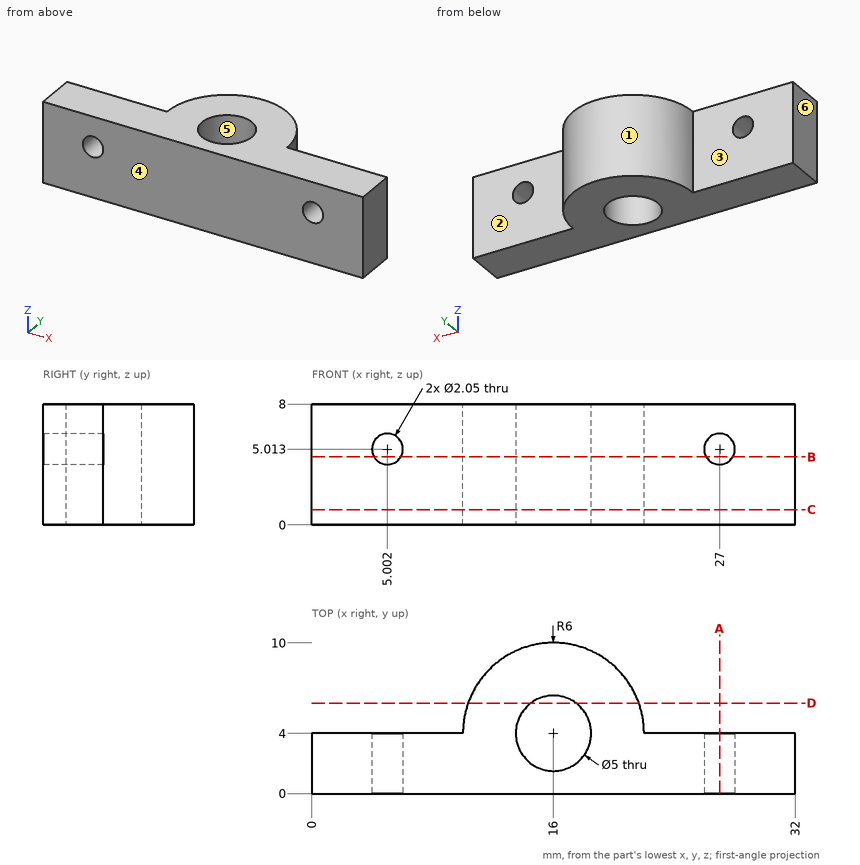
The figure shows three views and two pictorial views of one solid part (mm, origin at its lowest corner). Answer the questions. A direction names the side the tool comes from. Coordinates: 2 decimals unless noted, no trailing zeros. Loops run counter-clockwise (first coordinate to the right, second up) from the corner with the lowest first, then second, coordinate; pieces in that order, holes last. Notation, with made-up numbers: (-25.75, -12) - (4.25, -12) arc R21 cw to (4.25, 3) - close; hole circle Ø4 at (86, -25). An arc over 180 degrees is marked (long way). Write item = value, one per line.
1) Determine the mould class of the marked faces 4, 5 and 6 for opening direction X: pulls with the +X half, pulls with the -X half, needs draft (parallel to the pull), parting line crosses it, or undercut.
Responses:
face_4 = needs draft
face_5 = undercut
face_6 = pulls with the -X half
2) Section D-D (y = 6) is taken. Determine the outline of the cut face in (x, z).
Responses:
outline = (10.34, 0) - (14.5, 0) - (14.5, 8) - (10.34, 8) - close; (17.5, 0) - (21.66, 0) - (21.66, 8) - (17.5, 8) - close
3) Each of these flat-tipped pins is pushed along its axis until it touches: P1, Ø2.5, axis at x = 5, z = 5.01, coming from the +Y side; P2, Ø4, axis at x = 23.5, z = 5.5, coming from the +Y side (1 decimal). Where does it stop, or does it pass through?
Responses:
P1 = 4
P2 = 6.4
4) Section B-B (z = 4.5) is taken. Determine the outline of the cut face in (x, y).
Responses:
outline = (0, 0) - (4.11, 0) - (4.11, 4) - (0, 4) - close; (5.89, 0) - (26.11, 0) - (26.11, 4) - (22, 4) arc R6 ccw to (10, 4) - (5.89, 4) - close; (27.89, 0) - (32, 0) - (32, 4) - (27.89, 4) - close; hole circle Ø5 at (16, 4)
5) Which of the six approach directions +Z, -Z, +X, -X, +Y, -Y give full straight-line access (tool end or side, diameter ignored) to the marked faces 1, 2 and 3?
Responses:
face_1 = +Z, -Z, +Y
face_2 = +Z, -Z, +X, +Y
face_3 = +Z, -Z, -X, +Y
6) Section C-C (z = 1) is taken. Determine the outline of the cut face in (x, y), plus the area to 3 significant figures.
Responses:
outline = (0, 0) - (32, 0) - (32, 4) - (22, 4) arc R6 ccw to (10, 4) - (0, 4) - close; hole circle Ø5 at (16, 4)
area = 165 mm^2
7) Find the intervals of material crossed by line 1 along Z through (x, y) = (27, 1); line 2 along Y through (x, z) = (16, 3.25); line 3 along Y through (x, z) = (9, 4.25), in increasing order.
Responses:
line_1 = 0 to 3.99, 6.04 to 8
line_2 = 0 to 1.5, 6.5 to 10
line_3 = 0 to 4
8) Section A-A (x = 27) is taken. Determine the outline of the cut face in (y, z).
Responses:
outline = (0, 0) - (4, 0) - (4, 3.99) - (0, 3.99) - close; (0, 6.04) - (4, 6.04) - (4, 8) - (0, 8) - close
